Build history of the part. All positions in model axes, mm. A direction names the side the tool comes from. Round coordinates to 2 decimals unless told otherwise and drop trailing zeros. Write each loop counter-clockwise with the first axis right and the second up, starting at its lowest first coordinate (ties: lowest second). Pieces come first, ordered by that corner, then holes. Notation, with made-up numbers: (20.5, 23.25) - (30.5, 23.25) arc R21 ccw to (30.5, 38.25) - close; hole circle Ø6 at (-22.75, -9). An arc over 180 degrees is marked (long way). Write each question's results on one line, items separated by ' | '.
from build123d import *

# Parameters (mm, degrees)
SKETCH1_W               = 16.89
SKETCH1_H               = 15.16
BOSS_EXTRUDE1_DEPTH     = 29.8
CUT_EXTRUDE1_DEPTH      = 35.484541827
CUT_EXTRUDE1_DEPTH_BACK = 35.484541827
SKETCH2_W               = 14.55
SKETCH2_H               = 27.46
SKETCH3_R               = 3.25
BOSS_EXTRUDE2_DEPTH     = 21.2
CUT_EXTRUDE2_DEPTH      = 53.247243229
CUT_EXTRUDE2_DEPTH_BACK = 7.51
CUT_EXTRUDE3_DEPTH      = 32.887527734
CUT_EXTRUDE3_DEPTH_BACK = 32.887527734
SKETCH5_R               = 1.56
SKETCH6_R               = 2.675
BOSS_EXTRUDE3_DEPTH     = 7.41
FILLET1_R               = 2
SKETCH7_R               = 7.58
BOSS_EXTRUDE4_DEPTH     = 27.46
SKETCH8_R               = 0.805
BOSS_EXTRUDE7_DEPTH     = 5
FILLET2_R               = 0.5
CUT_EXTRUDE4_DEPTH      = 42.715278137
CUT_EXTRUDE4_DEPTH_BACK = 1.17
SKETCH9_R               = 1.35
BOSS_EXTRUDE8_START     = -8.58
SKETCH10_R              = 5.055
BOSS_EXTRUDE8_DEPTH     = 0.75


with BuildPart() as part:
    # Sketch1 → Boss-Extrude1 (new body)
    with BuildSketch(Plane(origin=(0, 0, 0), x_dir=(1, 0, 0), z_dir=(0, 1, 0))):
        Rectangle(SKETCH1_W, SKETCH1_H)
    extrude(amount=BOSS_EXTRUDE1_DEPTH)

    # Sketch2 → Cut-Extrude1 (cut, two sides: drawn at the far end of the back side and taken through both)
    with BuildSketch(Plane(origin=(0, 0, -7.58), x_dir=(-1, 0, 0), z_dir=(0, 0, -1)).offset(-CUT_EXTRUDE1_DEPTH_BACK)):
        with Locations((0, 14.9)):
            Rectangle(SKETCH2_W, SKETCH2_H)
    extrude(amount=CUT_EXTRUDE1_DEPTH + CUT_EXTRUDE1_DEPTH_BACK, mode=Mode.SUBTRACT)

    # Sketch3 → Boss-Extrude2 (add)
    with BuildSketch(Plane.XZ):
        with Locations(Location((0, 0, 0), (0, 0, 270))):
            Circle(SKETCH3_R)
    extrude(amount=BOSS_EXTRUDE2_DEPTH)

    # Sketch4 → Cut-Extrude2 (cut, two sides: drawn at the far end of the back side and taken through both)
    with BuildSketch(Plane.XZ.offset(21.2).offset(-CUT_EXTRUDE2_DEPTH_BACK)):
        with BuildLine():
            Line((-0.810006774, 3.147441664), (-0.810006774, -3.147441664))
            ThreePointArc((-0.810006774, -3.147441664), (-6.995e-06, -3.25), (0.809993226, -3.14744515))
            Line((0.809993226, -3.14744515), (0.809993226, 3.14744515))
            ThreePointArc((0.809993226, 3.14744515), (-6.995e-06, 3.25), (-0.810006774, 3.147441664))
        make_face()
    extrude(amount=CUT_EXTRUDE2_DEPTH + CUT_EXTRUDE2_DEPTH_BACK, mode=Mode.SUBTRACT)

    # Sketch5 → Cut-Extrude3 (cut, two sides: drawn at the far end of the back side and taken through both)
    with BuildSketch(Plane(origin=(0, 0, 0), x_dir=(0, 0, -1), z_dir=(1, 0, 0)).offset(-CUT_EXTRUDE3_DEPTH_BACK)):
        with Locations((0, -17.94)):
            Circle(SKETCH5_R)
    extrude(amount=CUT_EXTRUDE3_DEPTH + CUT_EXTRUDE3_DEPTH_BACK, mode=Mode.SUBTRACT)

    # Sketch6 → Boss-Extrude3 (add)
    with BuildSketch(Plane(origin=(0, 29.8, 0), x_dir=(1, 0, 0), z_dir=(0, 1, 0))):
        with Locations(Location((0, 0, 0), (0, 0, 270))):
            Circle(SKETCH6_R)
    extrude(amount=BOSS_EXTRUDE3_DEPTH)

    # Fillet1
    fillet1_edges = [part.edges().sort_by_distance(p)[0] for p in [
        (0, 37.21, -2.675),
    ]]
    fillet(fillet1_edges, radius=FILLET1_R)

    # Sketch7 → Boss-Extrude4 (add)
    with BuildSketch(Plane(origin=(0, 1.17, 0), x_dir=(1, 0, 0), z_dir=(0, 1, 0))):
        Circle(SKETCH7_R)
    extrude(amount=BOSS_EXTRUDE4_DEPTH)

    # Sketch8 → Boss-Extrude7 (add)
    with BuildSketch(Plane.XZ.offset(-28.63)):
        with Locations(Location((-0.85, -7.58, 0), (0, 0, 270))):
            Circle(SKETCH8_R)
        with Locations(Location((0.85, -7.58, 0), (0, 0, 270))):
            Circle(SKETCH8_R)
    extrude(amount=-BOSS_EXTRUDE7_DEPTH)

    # Fillet2
    fillet2_edges = [part.edges().sort_by_distance(p)[0] for p in [
        (-0.280779041, 28.63, -8.149220959),
        (-1.419220959, 28.63, -8.149220959),
        (0.280779041, 28.63, -8.149220959),
        (1.419220959, 28.63, -8.149220959),
    ]]
    fillet(fillet2_edges, radius=FILLET2_R)

    # Sketch9 → Cut-Extrude4 (cut, two sides: drawn at the far end of the back side and taken through both)
    with BuildSketch(Plane.ZY.offset(8.445).offset(-CUT_EXTRUDE4_DEPTH_BACK)):
        with Locations((4.34, 24.65)):
            Circle(SKETCH9_R)
        with Locations((-4.34, 5.02)):
            Circle(SKETCH9_R)
    extrude(amount=CUT_EXTRUDE4_DEPTH + CUT_EXTRUDE4_DEPTH_BACK, mode=Mode.SUBTRACT)

    # Sketch10 → Boss-Extrude8 (add)
    with BuildSketch(Plane.XZ.offset(21.2).offset(BOSS_EXTRUDE8_START)):
        with Locations(Location((0, 0, 0), (0, 0, 270))):
            Circle(SKETCH10_R)
    extrude(amount=-BOSS_EXTRUDE8_DEPTH)


solid = part.part
(1) Two-plate mould, pull along Y, no slides. Class faces 1 (the flat face through (0, -13.69, 0)), 2 (the flat face through (1, 33.63, -8)), 3 (the flat face through (-8.445, 15, 0)), 4 (the flat face through (-6, 1.17, 6)): released by +Y, released by -Y, zero draft, split by the parting line, or undercut.
Worked answers:
face 1: released by -Y | face 2: released by +Y | face 3: zero draft | face 4: undercut
(2) Slice it at C-C, the plane y = 22.5. Write the cut outline in (x, z) (3 decimals), and give its area (3 significant figures).
Worked answers:
outline: (-8.445, -7.58) - (-7.275, -7.58) - (-7.275, -2.129) arc R7.58 ccw to (7.275, -2.129) - (7.275, -7.58) - (8.445, -7.58) - (8.445, 7.58) - (7.275, 7.58) - (7.275, 2.129) arc R7.58 ccw to (-7.275, 2.129) - (-7.275, 7.58) - (-8.445, 7.58) - close | area: 214 mm2
(3) Tool access for faces 5 (the flat face through (6, 28.63, 6)), 6 (the flat face through (-1.1, -11.87, -3.3)), 7 (the flat face through (0.81, -16, 0)), 8 (the cylindrical face through (-2.61, 32.47, -0.58)): list every direction of +Z, -Z, +X, -X, +Y, -Y with a clear straight run to the whole face (end or side of a thin tool).
Worked answers:
face 5: +Z | face 6: none | face 7: +Z, -Z, -Y | face 8: +Y
(4) Flat gauge pins, fed straight in: pin 1 Ø1.3 at (x, z) = (-1, -7.5) entering from +Y; pin 2 Ø0.5 at (x, z) = (0, 1) entering from -Y; pin 3 Ø2 at (y, z) = (5.02, -4.34) entering from -X. Where does each tip first touch, or does it go through?
Worked answers:
pin 1: stops at y = 33.63 | pin 2: stops at y = -13.69 | pin 3: stops at x = -6.8
(5) Slice it at B-B, the plane y = 5.02. Write the cut outline in (x, z) (3 decimals), and give its area (3 significant figures).
Worked answers:
outline: (-8.445, -7.58) - (-7.275, -7.58) - (-7.275, -5.69) - (-8.445, -5.69) - close; (-8.445, -2.99) - (-7.275, -2.99) - (-7.275, -2.129) arc R7.58 ccw to (7.275, -2.129) - (7.275, -7.58) - (8.445, -7.58) - (8.445, 7.58) - (7.275, 7.58) - (7.275, 2.129) arc R7.58 ccw to (-7.275, 2.129) - (-7.275, 7.58) - (-8.445, 7.58) - close | area: 211 mm2
(6) Slice it at A-A, the plane z = -4.34. Write the cut outline in (x, y) (3 decimals).
Worked answers:
outline: (-8.445, 0) - (8.445, 0) - (8.445, 29.8) - (-8.445, 29.8) - (-8.445, 6.37) - (-7.275, 6.37) - (-7.275, 28.63) - (-6.215, 28.63) - (-6.215, 1.17) - (-7.275, 1.17) - (-7.275, 3.67) - (-8.445, 3.67) - close; (-2.592, -12.62) - (2.592, -12.62) - (2.592, -11.87) - (-2.592, -11.87) - close; hole (6.215, 1.17) - (7.275, 1.17) - (7.275, 28.63) - (6.215, 28.63) - close
(7) Drill centre lines: probe 1 along Y at (x, z) = (-8, -4.34); probe 2 along X at (y, z) = (6, 4.5) (3 decimals); probe 3 along Y at (x, z) = (-1, 4.75). Where is each one in solid material? Low to high. Write a range as [from, to].
Worked answers:
probe 1: y = [0, 3.67], [6.37, 29.8] | probe 2: x = [-8.445, -7.275], [-6.1, 6.1], [7.275, 8.445] | probe 3: y = [-12.62, -11.87], [0, 29.8]
